Model file for the job. Use its own axes, mm. A direction names the side the tool comes from. Round coordinates to 2 decimals unless told otherwise and drop trailing zeros. Loops run counter-clockwise (first coordinate to the right, second up) from the corner with the lowest first, then second, coordinate; pieces in that order, holes last. Notation, with made-up numbers: (74, -37.75) - (89, -37.75) arc R31 cw to (89, 1.25) - close; hole circle Ø8 at (20.25, -35.5). An arc over 180 degrees is marked (long way). Answer as a JSON object with one key per item and string values.
Autodesk Inventor part; units mm, degrees
ref_plane "Work Plane3" through (0, 0, 1000) normal (0, 0, 1) x (1, 0, 0)
ref_plane "YZ Plane" through (0, 0, 0) normal (1, 0, 0) x (0, 1, 0)
ref_plane "XZ Plane" through (0, 0, 0) normal (0, 1, 0) x (-1, 0, 0)
sketch "Sketch1" plane through (0, 0, 0) normal (0, 1, 0) x (-1, 0, 0)
  line L0 (-12, 14) -> (12, 14) construction
  line L1 (14, 12) -> (14, -12) construction
  line L2 (12, -14) -> (-12, -14) construction
  line L3 (-14, -12) -> (-14, 12) construction
  line L4 (-14, 14) -> (14, -14) construction
  line L5 (14, 14) -> (-14, -14) construction
  arc A0 (14, 12) -> (12, 14) centre (12, 12) ccw construction
  arc A1 (12, -14) -> (14, -12) centre (12, -12) ccw construction
  arc A2 (-14, -12) -> (-12, -14) centre (-12, -12) ccw construction
  arc A3 (-12, 14) -> (-14, 12) centre (-12, 12) ccw construction
  line L6 (-12, -15) -> (12, -15)
  arc A4 (12, -15) -> (15, -12) centre (12, -12) ccw
  line L7 (15, -12) -> (15, 12)
  arc A5 (15, 12) -> (12, 15) centre (12, 12) ccw
  line L8 (12, 15) -> (-12, 15)
  arc A6 (-12, 15) -> (-15, 12) centre (-12, 12) ccw
  line L9 (-15, 12) -> (-15, -12)
  arc A7 (-15, -12) -> (-12, -15) centre (-12, -12) ccw
  line L10 (13, -12) -> (13, 12)
  arc A8 (13, 12) -> (12, 13) centre (12, 12) ccw
  line L11 (12, 13) -> (-12, 13)
  arc A9 (-12, 13) -> (-13, 12) centre (-12, 12) ccw
  line L12 (-13, 12) -> (-13, -12)
  arc A10 (-13, -12) -> (-12, -13) centre (-12, -12) ccw
  line L13 (-12, -13) -> (12, -13)
  arc A11 (12, -13) -> (13, -12) centre (12, -12) ccw
  point P0 (0, 0)
  point P1 (0, 0)
  point P2 (0, 0)
  dimension "d10" = 2
  dimension "depth" = 30
  dimension "width" = 30
  dimension "thickness" = 2
sketch "Sketch3" plane through (0, 0, 0) normal (1, 0, 0) x (0, 1, 0)
  line L0 (0, 0) -> (0, 2000) construction
  arc A0 (0, 0) -> (0, 2000) centre (0, 1000) ccw
  line L1 (0, -400) -> (0, 2400)
  line L2 (-200, 0) -> (1200, 0)
  dimension "d30" = 2000
  dimension "d31" = 1000
sweep "Sweep1" add profiles "Sketch1" path "Sketch3" path curves A0
sketch "Sketch5" plane through (-15, 0, 1000) normal (-1, 0, 0) x (0, 0, 1)
  arc A0 (1000, 0) -> (-1000, 0) centre (0, 0) ccw construction
  line L0 (-1012, 0) -> (-988, 0)
  line L1 (1012, 0) -> (988, 0)
  point P0 (-1000, 0)
  point P1 (-998.7492, 50)
  point P2 (-995.0016, 99.8594)
  point P3 (1000, 0)
  point P4 (998.7492, 50)
  point P5 (995.0016, 99.8594)
  dimension "d46" = 50
  dimension "d51" = 50
  dimension "d52" = 50
  dimension "d53" = 50
hole "Hole3" at (-15, 50, 1.2508) at (-15, 99.8594, 4.9984) at (-15, 50, 1998.7492) at (-15, 99.8594, 1995.0016) direction (1, 0, 0) diameter 9 depth 20.2 tip angle 118
ref_plane "Work Plane3" through (0, 0, 1000) normal (0, 0, 1) x (1, 0, 0)
equation "\"d10\" = thickness"
equation "\"d31\" = 0.5 * d30"
properties part number "Luk R2000 podest" material "Steel"
1) Tool access for faces 1 (the cylindrical face through (0.168, 1012.755, 977.725)), 2 (the cylindrical face through (0.17, 984.76, 978.34)): list every direction of +Z, -Z, +X, -X, +Y, -Y with a clear straight run to the whole face (end or side of a thin tool).
Values follow:
{"face 1": "none", "face 2": "+X, -X, -Y"}
2) Probe probe 1 along Z at (x, y) = (-14.6, 50); probe 2 along Z at (x, y) = (-13.9, 50); probe 3 along Y at (x, z) = (-1, 990). List the from-to ranges inside material, lowest first.
Values follow:
{"probe 1": "-12.26 to -3.25, 5.75 to 14.76, 1985.24 to 1994.25, 2003.25 to 2012.26", "probe 2": "-13.09 to -3.25, 5.75 to 15.59, 1984.41 to 1994.25, 2003.25 to 2013.09", "probe 3": "984.95 to 986.95, 1012.95 to 1014.95"}
3) Drop flat-ended pins along their axis: P1, Ø8, axis at x = -9, y = 234.5, coming from the +Z side; P2, Ø1.5, axis at x = -6, y = 179.5, coming from the -Z side; P3, Ø3, axis at x = -10.5, y = 211.5, coming from the +Z side. Give the stop position or say it passes through.
Values follow:
{"P1": "z = 1988.48", "P2": "z = 0.86", "P3": "z = 1993.04"}
4) Slice it at A-A on x = -3. List the corners of the cut face in (y, z), then the cut area to 3 significant figures.
Values follow:
{"outline": "(0, -15) arc R1015 ccw to (0, 2015) - (0, 2013) arc R1013 cw to (0, -13) - close; (0, 13) arc R987 ccw to (0, 1987) - (0, 1985) arc R985 cw to (0, 15) - close", "area": "12,600 mm²"}
5) Slice it at B-B on z = 1000. List the corners of the cut face in (x, y).
Values follow:
{"outline": "(-15, 988) arc R3 ccw to (-12, 985) - (12, 985) arc R3 ccw to (15, 988) - (15, 1012) arc R3 ccw to (12, 1015) - (-12, 1015) arc R3 ccw to (-15, 1012) - close; hole (-13, 988) arc R1 ccw to (-12, 987) - (12, 987) arc R1 ccw to (13, 988) - (13, 1012) arc R1 ccw to (12, 1013) - (-12, 1013) arc R1 ccw to (-13, 1012) - close"}
6) Two-plate mould, pull along Y, no slides. Class faces 3 (the cylindrical face through (-0.168, 1014.755, 1022.319)), 4 (the flat face through (15, 996, 995)), 5 (the flat face through (-13, 996, 995)): pulls with the +Y half, pulls with the -Y half, needs draft (parallel to the pull), parting line crosses it, or undercut.
Values follow:
{"face 3": "pulls with the +Y half", "face 4": "needs draft", "face 5": "undercut"}
